from build123d import *

# Parameters (mm, degrees)
F0_R     = 60
F1_DEPTH = 35
F2_R     = 60
F3_DEPTH = 27
F4_R     = 3.75
F5_DEPTH = 44.75074


with BuildPart() as f1:
    # F0 (on Right) → F1 (new body)
    with BuildSketch(Plane.YZ):
        Circle(F0_R)
        Polygon((0, 13.2790561914), (11.5, 6.6395280957), (11.5, -6.6395280957), (0, -13.2790561914), (-11.5, -6.6395280957), (-11.5, 6.6395280957), align=None, mode=Mode.SUBTRACT)
    extrude(amount=F1_DEPTH)

    # F2 (on face) → F3 (cut)
    with BuildSketch(Plane.YZ.offset(35)):
        Circle(F2_R)
        Polygon((0, 15.0111069989), (13, 7.5055534995), (13, -7.5055534995), (0, -15.0111069989), (-13, -7.5055534995), (-13, 7.5055534995), align=None, mode=Mode.SUBTRACT)
    extrude(amount=-F3_DEPTH, mode=Mode.SUBTRACT)

    # F4 (on face) → F5 (cut)
    with BuildSketch(Plane(origin=(0, 13, 0), x_dir=(-1, 0, 0), z_dir=(0, 1, 0))):
        with Locations((-17.5, 0)):
            Circle(F4_R)
    extrude(amount=-F5_DEPTH, mode=Mode.SUBTRACT)


solid = f1.part
Input: part model. Units: mm. Frame: model coordinates. A direction names the side the tool comes from. Round coordinates to 2 decimals unless told otherwise and drop trailing zeros. Order: outer loops, then holes, each group sorted by start corner. A loop starts at its lowest first (then second) coordinate and runs counter-clockwise, first axis right, second up. Notation, with made-up numbers: (43, 35.5) - (82, 35.5) arc R25 cw to (82, 58.5) - close; hole circle Ø11 at (72, -7.5). An arc over 180 degrees is marked (long way). Answer as a JSON object with one key per item and string values. Group by question number.
(1) Pin query (flat end, axial travel): P1, Ø7.5, axis at x = 18.5, z = 2.5, coming from the +Y side; P2, Ø10, axis at x = 17.5, z = 0, coming from the -Y side; P3, Ø1, axis at y = 23.5, z = -10.5, coming from the +X side. Return the tip coordinate at first contact, or that it passes through.
(2) Reachability of faces 4 (the face through (17.255, 5.67, 10.006)), 5 (the face through (22, -13, 0)), 6 (the face through (21.69, 6.41, 11.31)) from +Z, -Z, +X, -X, +Y, -Y: full face, straight path, thin tool, end or side. Return the list, or none.
(3) Material intervals for probe 1 along Y at (x, z) = (16, 4); probe 2 along X at (y, z) = (42.5, -23.5); probe 3 along Z at (x, y) = (17.5, -12.4), sorted ascending. Write a range as from..to.
(4) Draft query along Y for faces 1 (the face through (21.7, 6.6, -11.2)), 2 (the face through (17.255, 5.83, -9.913)), 3 (the face through (8, -14, 1)). Return one class per face: released by +Y, released by -Y, zero draft, split by the parting line, or undercut.
(5) Cut plane D-D (x = 17.5). Return loops of the section in (y, z), then the cut area to 3 significant figures.
(6) Cut plane A-A (z = 0). Return loops of the section in (x, y).
(7) Cut plane C-C (y = 8). Return loops of the section in (x, z), then the cut area to 3 significant figures.
(8) Cut plane B-B (x = 33). Return loops of the section in (y, z).
Here are the results:
{
 "1": {"P1": "stops at y = 13", "P2": "stops at y = -13", "P3": "stops at x = 8"},
 "2": {"face 4": "+X, -X", "face 5": "+Z, -Z, +X, -Y", "face 6": "+Z, +X, +Y"},
 "3": {"probe 1": "y = -13..-11.5, 11.5..13", "probe 2": "x = 0..8", "probe 3": "z = -7.85..-3.75, 3.75..7.85"},
 "4": {"face 1": "released by +Y", "face 2": "undercut", "face 3": "zero draft"},
 "5": {"outline": "(-13, -7.51) - (0, -15.01) - (13, -7.51) - (13, -3.75) - (11.5, -3.75) - (11.5, -6.64) - (0, -13.28) - (-11.5, -6.64) - (-11.5, -3.75) - (-13, -3.75) - close; (-13, 3.75) - (-11.5, 3.75) - (-11.5, 6.64) - (0, 13.28) - (11.5, 6.64) - (11.5, 3.75) - (13, 3.75) - (13, 7.51) - (0, 15.01) - (-13, 7.51) - close", "area": "105 mm^2"},
 "6": {"outline": "(0, -60) - (8, -60) - (8, -13) - (13.75, -13) - (13.75, -11.5) - (0, -11.5) - close; (0, 11.5) - (13.75, 11.5) - (13.75, 13) - (8, 13) - (8, 60) - (0, 60) - close; (21.25, -13) - (35, -13) - (35, -11.5) - (21.25, -11.5) - close; (21.25, 11.5) - (35, 11.5) - (35, 13) - (21.25, 13) - close"},
 "7": {"outline": "(0, -59.46) - (8, -59.46) - (8, -10.39) - (35, -10.39) - (35, -8.66) - (0, -8.66) - close; (0, 8.66) - (35, 8.66) - (35, 10.39) - (8, 10.39) - (8, 59.46) - (0, 59.46) - close", "area": "906 mm^2"},
 "8": {"outline": "(-13, -7.51) - (0, -15.01) - (13, -7.51) - (13, 7.51) - (0, 15.01) - (-13, 7.51) - close; hole (-11.5, -6.64) - (0, -13.28) - (11.5, -6.64) - (11.5, 6.64) - (0, 13.28) - (-11.5, 6.64) - close"}
}
